Here's how the part is built. I have some questions about the finished solid (model axes, mm). A direction names the side the tool comes from. Round coordinates to 2 decimals unless told otherwise and drop trailing zeros. Write each loop counter-clockwise with the first axis right and the second up, starting at its lowest first coordinate (ties: lowest second). Pieces come first, ordered by that corner, then holes. Notation, with made-up numbers: (59, 68) -> (70, 68) arc R36 cw to (70, 105) -> close; hole circle Ø5 at (85, -22.5). An arc over 180 degrees is marked (long way). Answer as CSV lines item,"result".
```python
from build123d import *

# Parameters (mm, degrees)
F0_R     = 17.2924664606
F0_R_2   = 1.65
F0_R_3   = 9.7924664606
F1_DEPTH = 2
F2_DEPTH = 5
F3_SIZE  = 1.5


# Not quite as in the source:
# - a fillet or chamfer that OpenCascade refuses, or shapes differently, is made with other operations: its cross-section is extruded or revolved along the edge and cut away or added


with BuildPart() as f1:
    # F0 (on Front) → F1 (new body)
    with BuildSketch(Plane.XZ):
        Circle(F0_R)
        with Locations((-13.4424664606, 0)):
            Circle(F0_R_2, mode=Mode.SUBTRACT)
        Circle(F0_R_3, mode=Mode.SUBTRACT)
        with Locations((13.4424664606, 0)):
            Circle(F0_R_2, mode=Mode.SUBTRACT)
        Circle(F0_R_3)
        with BuildLine():
            ThreePointArc((8.2924664606, 0), (7.7650793743, -2.9100759974), (6.25, -5.45))
            ThreePointArc((6.25, -5.45), (0, -8.2924664606), (-6.25, -5.45))
            ThreePointArc((-6.25, -5.45), (-8.2924664606, 0), (-6.25, 5.45))
            ThreePointArc((-6.25, 5.45), (0, 8.2924664606), (6.25, 5.45))
            ThreePointArc((6.25, 5.45), (7.7650793743, 2.9100759974), (8.2924664606, 0))
        make_face(mode=Mode.SUBTRACT)
        with BuildLine():
            ThreePointArc((-6.25, 5.45), (-8.2924664606, 0), (-6.25, -5.45))
            Line((-6.25, -5.45), (-6.25, 5.45))
        make_face()
        with BuildLine():
            Line((-6.25, 5.45), (6.25, 5.45))
            ThreePointArc((6.25, 5.45), (0, 8.2924664606), (-6.25, 5.45))
        make_face()
        with BuildLine():
            Line((6.25, 5.45), (6.25, -5.45))
            ThreePointArc((6.25, -5.45), (7.7650793743, -2.9100759974), (8.2924664606, 0))
            ThreePointArc((8.2924664606, 0), (7.7650793743, 2.9100759974), (6.25, 5.45))
        make_face()
        with BuildLine():
            ThreePointArc((-6.25, -5.45), (0, -8.2924664606), (6.25, -5.45))
            Line((6.25, -5.45), (-6.25, -5.45))
        make_face()
    extrude(amount=-F1_DEPTH)

    # F0 (on Front) → F2 (join)
    with BuildSketch(Plane.XZ):
        Circle(F0_R_3)
        with BuildLine():
            ThreePointArc((8.2924664606, 0), (7.7650793743, -2.9100759974), (6.25, -5.45))
            ThreePointArc((6.25, -5.45), (0, -8.2924664606), (-6.25, -5.45))
            ThreePointArc((-6.25, -5.45), (-8.2924664606, 0), (-6.25, 5.45))
            ThreePointArc((-6.25, 5.45), (0, 8.2924664606), (6.25, 5.45))
            ThreePointArc((6.25, 5.45), (7.7650793743, 2.9100759974), (8.2924664606, 0))
        make_face(mode=Mode.SUBTRACT)
        with BuildLine():
            ThreePointArc((-6.25, 5.45), (-8.2924664606, 0), (-6.25, -5.45))
            Line((-6.25, -5.45), (-6.25, 5.45))
        make_face()
        with BuildLine():
            Line((-6.25, 5.45), (6.25, 5.45))
            ThreePointArc((6.25, 5.45), (0, 8.2924664606), (-6.25, 5.45))
        make_face()
        with BuildLine():
            Line((6.25, 5.45), (6.25, -5.45))
            ThreePointArc((6.25, -5.45), (7.7650793743, -2.9100759974), (8.2924664606, 0))
            ThreePointArc((8.2924664606, 0), (7.7650793743, 2.9100759974), (6.25, 5.45))
        make_face()
        with BuildLine():
            ThreePointArc((-6.25, -5.45), (0, -8.2924664606), (6.25, -5.45))
            Line((6.25, -5.45), (-6.25, -5.45))
        make_face()
    extrude(amount=F2_DEPTH)

    # F3
    f3_edges = [f1.edges().sort_by_distance(p)[0] for p in [
        (11.792466, 2, 0),
        (-15.092466, 2, 0),
    ]]
    chamfer(f3_edges, length=F3_SIZE)

    # F4: fillet of radius 1.8 on 1 edges, made by hand

    # F4_s1 → F4_t2 (revolve, cut)
    with BuildSketch(Plane.XY):
        with BuildLine():
            ThreePointArc((15.4924664606, 2), (16.7652586667, 1.4727922061), (17.2924664606, 0.2))
            Line((17.2924664606, 0.2), (17.2924664606, 2))
            Line((17.2924664606, 2), (15.4924664606, 2))
        make_face()
    revolve(axis=Axis((0, 2, 0), (0, -1, 0)), mode=Mode.SUBTRACT)


solid = f1.part
```
1. For pin 1 Ø1.5 at (x, z) = (-3, 13) entering from -Y; pin 2 Ø2 at (x, z) = (13.44, 0) entering from -Y; pin 3 Ø3.5 at (y, z) = (-2.5, 0.5) entering from +X; pin 4 Ø2 at (x, y) = (9, -2) entering from -Z, each with a flat end and sliding along its axis, tell me the tip position at first contact or that it passes through.
Numbers:
pin 1,"stops at y = 0"
pin 2,"passes through"
pin 3,"stops at x = 9.79"
pin 4,"stops at z = -5.65"
2. If I drill on line 1 (X direction, y = 1.5, z = -2); line 2 (Y direction, x = 1, z = 15); line 3 (X direction, y = -2.5, z = -3.5), over which ranges is the centre line in solid material (lowest first)?
Numbers:
line 1,"x = -16.62 to -15.18, -11.7 to -6.25, 6.25 to 11.7, 15.18 to 16.62"
line 2,"y = 0 to 2"
line 3,"x = -9.15 to -6.25, 6.25 to 9.15"
3. Suppose I cut it at A-A on x = 0. Please give me the cut outline in (y, z), and give its area (3 significant figures).
Numbers:
outline,"(-5, -9.79) -> (0, -9.79) -> (0, -17.29) -> (0.2, -17.29) arc R1.8 ccw to (2, -15.49) -> (2, -5.45) -> (-5, -5.45) -> close; (-5, 5.45) -> (2, 5.45) -> (2, 15.49) arc R1.8 ccw to (0.2, 17.29) -> (0, 17.29) -> (0, 9.79) -> (-5, 9.79) -> close"
area,"89.4 mm^2"
4. Suppose I cut it at B-B on z = 0. Please give me the cut outline in (x, y), and give its area (3 significant figures).
Numbers:
outline,"(-17.29, 0) -> (-15.09, 0) -> (-15.09, 0.5) -> (-16.37, 1.77) arc R1.8 ccw to (-17.29, 0.2) -> close; (-11.79, 0) -> (-9.79, 0) -> (-9.79, -5) -> (-6.25, -5) -> (-6.25, 2) -> (-10.29, 2) -> (-11.79, 0.5) -> close; (6.25, -5) -> (9.79, -5) -> (9.79, 0) -> (11.79, 0) -> (11.79, 0.5) -> (10.29, 2) -> (6.25, 2) -> close; (15.09, 0) -> (17.29, 0) -> (17.29, 0.2) arc R1.8 ccw to (16.37, 1.77) -> (15.09, 0.5) -> close"
area,"60.7 mm^2"
5. If we mould it in two halves opening along X, with no side actions, what happens to faces 1 (the face through (6.4, -5, 0.1)), 2 (the face through (-15.09, 0.25, 0.07)), 3 (the face through (-2.12, -2.46, -9.56))? For each: released by +X, released by -X, zero draft, split by the parting line, or undercut.
Numbers:
face 1,"zero draft"
face 2,"undercut"
face 3,"split by the parting line"
6. On a 3-axis mill with a long thin cutter (end or side, diameter ignored), from which of +Z, -Z, +X, -X, +Y, -Y can I reach the whole of each face in a straight line? I mean faces 4 (the face through (7, 2, 0)), 5 (the face through (6.25, -1, 0)), 6 (the face through (7.4, 0, -7.4)). Say none if no direction works.
Numbers:
face 4,"+Z, -Z, +X, -X, +Y"
face 5,"+Y, -Y"
face 6,"-Y"
